```python
from build123d import *

# Parameters (mm, degrees)
F0_R     = 1.778
F1_DEPTH = 3.5
F2_DEPTH = 4


with BuildPart() as f1:
    # F0 (on Top) → F1 (new body)
    with BuildSketch(Plane.XY):
        with BuildLine():
            ThreePointArc((0, 5), (1.464466, 1.464466), (5, 0))
            Line((5, 0), (75, 0))
            Line((75, 0), (145, 0))
            ThreePointArc((145, 0), (148.535534, 1.464466), (150, 5))
            Line((150, 5), (150, 10))
            Line((150, 10), (150, 22.333333))
            Line((150, 22.333333), (150, 32.333333))
            Line((150, 32.333333), (150, 44.666667))
            Line((150, 44.666667), (150, 44.792384))
            Line((150, 44.792384), (150, 54.666667))
            Line((150, 54.666667), (150, 67))
            Line((150, 67), (150, 72))
            ThreePointArc((150, 72), (148.535534, 75.535534), (145, 77))
            Line((145, 77), (75, 77))
            Line((75, 77), (5, 77))
            ThreePointArc((5, 77), (1.464466, 75.535534), (0, 72))
            Line((0, 72), (0, 67))
            Line((0, 67), (0, 54.666667))
            Line((0, 54.666667), (0, 44.792384))
            Line((0, 44.792384), (0, 44.666667))
            Line((0, 44.666667), (0, 32.333333))
            Line((0, 32.333333), (0, 22.333333))
            Line((0, 22.333333), (0, 10))
            Line((0, 10), (0, 5))
        make_face()
        with Locations((7.5, 5)):
            Circle(F0_R, mode=Mode.SUBTRACT)
        with Locations((62, 5)):
            Circle(F0_R, mode=Mode.SUBTRACT)
        with BuildLine():
            Line((60.399714, 10), (18.611655, 10))
            ThreePointArc((18.611655, 10), (15.076121, 11.464466), (13.611655, 15))
            Line((13.611655, 15), (13.611655, 17.333333))
            ThreePointArc((13.611655, 17.333333), (15.076121, 20.868867), (18.611655, 22.333333))
            Line((18.611655, 22.333333), (60.399714, 22.333333))
            ThreePointArc((60.399714, 22.333333), (63.935248, 20.868867), (65.399714, 17.333333))
            Line((65.399714, 17.333333), (65.399714, 15))
            ThreePointArc((65.399714, 15), (63.935248, 11.464466), (60.399714, 10))
        make_face(mode=Mode.SUBTRACT)
        with Locations((7.5, 27.333333)):
            Circle(F0_R, mode=Mode.SUBTRACT)
        with Locations((62, 27.333333)):
            Circle(F0_R, mode=Mode.SUBTRACT)
        with Locations((88, 5)):
            Circle(F0_R, mode=Mode.SUBTRACT)
        with BuildLine():
            ThreePointArc((131.388345, 22.333333), (134.923879, 20.868867), (136.388345, 17.333333))
            Line((136.388345, 17.333333), (136.388345, 15))
            ThreePointArc((136.388345, 15), (134.923879, 11.464466), (131.388345, 10))
            Line((131.388345, 10), (89.600286, 10))
            ThreePointArc((89.600286, 10), (86.064752, 11.464466), (84.600286, 15))
            Line((84.600286, 15), (84.600286, 17.333333))
            ThreePointArc((84.600286, 17.333333), (86.064752, 20.868867), (89.600286, 22.333333))
            Line((89.600286, 22.333333), (131.388345, 22.333333))
        make_face(mode=Mode.SUBTRACT)
        with Locations((142.5, 5)):
            Circle(F0_R, mode=Mode.SUBTRACT)
        with Locations((88, 27.333333)):
            Circle(F0_R, mode=Mode.SUBTRACT)
        with Locations((142.5, 27.333333)):
            Circle(F0_R, mode=Mode.SUBTRACT)
        with Locations((7.5, 49.666667)):
            Circle(F0_R, mode=Mode.SUBTRACT)
        with BuildLine():
            Line((60.399714, 32.333333), (18.611655, 32.333333))
            ThreePointArc((18.611655, 32.333333), (15.076121, 33.797799), (13.611655, 37.333333))
            Line((13.611655, 37.333333), (13.611655, 39.792384))
            ThreePointArc((13.611655, 39.792384), (15.076121, 43.327917), (18.611655, 44.792384))
            Line((18.611655, 44.792384), (60.399714, 44.792384))
            ThreePointArc((60.399714, 44.792384), (63.935248, 43.327917), (65.399714, 39.792384))
            Line((65.399714, 39.792384), (65.399714, 37.333333))
            ThreePointArc((65.399714, 37.333333), (63.935248, 33.797799), (60.399714, 32.333333))
        make_face(mode=Mode.SUBTRACT)
        with Locations((62, 49.666667)):
            Circle(F0_R, mode=Mode.SUBTRACT)
        with Locations((7.5, 72)):
            Circle(F0_R, mode=Mode.SUBTRACT)
        with BuildLine():
            Line((60.399714, 54.666667), (18.611655, 54.666667))
            ThreePointArc((18.611655, 54.666667), (15.076121, 56.131133), (13.611655, 59.666667))
            Line((13.611655, 59.666667), (13.611655, 62))
            ThreePointArc((13.611655, 62), (15.076121, 65.535534), (18.611655, 67))
            Line((18.611655, 67), (60.399714, 67))
            ThreePointArc((60.399714, 67), (63.935248, 65.535534), (65.399714, 62))
            Line((65.399714, 62), (65.399714, 59.666667))
            ThreePointArc((65.399714, 59.666667), (63.935248, 56.131133), (60.399714, 54.666667))
        make_face(mode=Mode.SUBTRACT)
        with Locations((62, 72)):
            Circle(F0_R, mode=Mode.SUBTRACT)
        with BuildLine():
            Line((89.600286, 44.792384), (131.388345, 44.792384))
            ThreePointArc((131.388345, 44.792384), (134.923879, 43.327917), (136.388345, 39.792384))
            Line((136.388345, 39.792384), (136.388345, 37.333333))
            ThreePointArc((136.388345, 37.333333), (134.923879, 33.797799), (131.388345, 32.333333))
            Line((131.388345, 32.333333), (89.600286, 32.333333))
            ThreePointArc((89.600286, 32.333333), (86.064752, 33.797799), (84.600286, 37.333333))
            Line((84.600286, 37.333333), (84.600286, 39.792384))
            ThreePointArc((84.600286, 39.792384), (86.064752, 43.327917), (89.600286, 44.792384))
        make_face(mode=Mode.SUBTRACT)
        with Locations((88, 49.666667)):
            Circle(F0_R, mode=Mode.SUBTRACT)
        with Locations((142.5, 49.666667)):
            Circle(F0_R, mode=Mode.SUBTRACT)
        with BuildLine():
            ThreePointArc((131.388345, 67), (134.923879, 65.535534), (136.388345, 62))
            Line((136.388345, 62), (136.388345, 59.666667))
            ThreePointArc((136.388345, 59.666667), (134.923879, 56.131133), (131.388345, 54.666667))
            Line((131.388345, 54.666667), (89.600286, 54.666667))
            ThreePointArc((89.600286, 54.666667), (86.064752, 56.131133), (84.600286, 59.666667))
            Line((84.600286, 59.666667), (84.600286, 62))
            ThreePointArc((84.600286, 62), (86.064752, 65.535534), (89.600286, 67))
            Line((89.600286, 67), (131.388345, 67))
        make_face(mode=Mode.SUBTRACT)
        with Locations((88, 72)):
            Circle(F0_R, mode=Mode.SUBTRACT)
        with Locations((142.5, 72)):
            Circle(F0_R, mode=Mode.SUBTRACT)
    extrude(amount=F1_DEPTH)

    # F0 (on Top) → F2 (join)
    with BuildSketch(Plane.XY):
        with BuildLine():
            ThreePointArc((0, 5), (1.464466, 1.464466), (5, 0))
            Line((5, 0), (75, 0))
            Line((75, 0), (145, 0))
            ThreePointArc((145, 0), (148.535534, 1.464466), (150, 5))
            Line((150, 5), (150, 10))
            Line((150, 10), (150, 22.333333))
            Line((150, 22.333333), (150, 32.333333))
            Line((150, 32.333333), (150, 44.666667))
            Line((150, 44.666667), (150, 44.792384))
            Line((150, 44.792384), (150, 54.666667))
            Line((150, 54.666667), (150, 67))
            Line((150, 67), (150, 72))
            ThreePointArc((150, 72), (148.535534, 75.535534), (145, 77))
            Line((145, 77), (75, 77))
            Line((75, 77), (5, 77))
            ThreePointArc((5, 77), (1.464466, 75.535534), (0, 72))
            Line((0, 72), (0, 67))
            Line((0, 67), (0, 54.666667))
            Line((0, 54.666667), (0, 44.792384))
            Line((0, 44.792384), (0, 44.666667))
            Line((0, 44.666667), (0, 32.333333))
            Line((0, 32.333333), (0, 22.333333))
            Line((0, 22.333333), (0, 10))
            Line((0, 10), (0, 5))
        make_face()
        with Locations((7.5, 5)):
            Circle(F0_R, mode=Mode.SUBTRACT)
        with Locations((62, 5)):
            Circle(F0_R, mode=Mode.SUBTRACT)
        with BuildLine():
            Line((60.399714, 10), (18.611655, 10))
            ThreePointArc((18.611655, 10), (15.076121, 11.464466), (13.611655, 15))
            Line((13.611655, 15), (13.611655, 17.333333))
            ThreePointArc((13.611655, 17.333333), (15.076121, 20.868867), (18.611655, 22.333333))
            Line((18.611655, 22.333333), (60.399714, 22.333333))
            ThreePointArc((60.399714, 22.333333), (63.935248, 20.868867), (65.399714, 17.333333))
            Line((65.399714, 17.333333), (65.399714, 15))
            ThreePointArc((65.399714, 15), (63.935248, 11.464466), (60.399714, 10))
        make_face(mode=Mode.SUBTRACT)
        with Locations((7.5, 27.333333)):
            Circle(F0_R, mode=Mode.SUBTRACT)
        with Locations((62, 27.333333)):
            Circle(F0_R, mode=Mode.SUBTRACT)
        with Locations((88, 5)):
            Circle(F0_R, mode=Mode.SUBTRACT)
        with BuildLine():
            ThreePointArc((131.388345, 22.333333), (134.923879, 20.868867), (136.388345, 17.333333))
            Line((136.388345, 17.333333), (136.388345, 15))
            ThreePointArc((136.388345, 15), (134.923879, 11.464466), (131.388345, 10))
            Line((131.388345, 10), (89.600286, 10))
            ThreePointArc((89.600286, 10), (86.064752, 11.464466), (84.600286, 15))
            Line((84.600286, 15), (84.600286, 17.333333))
            ThreePointArc((84.600286, 17.333333), (86.064752, 20.868867), (89.600286, 22.333333))
            Line((89.600286, 22.333333), (131.388345, 22.333333))
        make_face(mode=Mode.SUBTRACT)
        with Locations((142.5, 5)):
            Circle(F0_R, mode=Mode.SUBTRACT)
        with Locations((88, 27.333333)):
            Circle(F0_R, mode=Mode.SUBTRACT)
        with Locations((142.5, 27.333333)):
            Circle(F0_R, mode=Mode.SUBTRACT)
        with Locations((7.5, 49.666667)):
            Circle(F0_R, mode=Mode.SUBTRACT)
        with BuildLine():
            Line((60.399714, 32.333333), (18.611655, 32.333333))
            ThreePointArc((18.611655, 32.333333), (15.076121, 33.797799), (13.611655, 37.333333))
            Line((13.611655, 37.333333), (13.611655, 39.792384))
            ThreePointArc((13.611655, 39.792384), (15.076121, 43.327917), (18.611655, 44.792384))
            Line((18.611655, 44.792384), (60.399714, 44.792384))
            ThreePointArc((60.399714, 44.792384), (63.935248, 43.327917), (65.399714, 39.792384))
            Line((65.399714, 39.792384), (65.399714, 37.333333))
            ThreePointArc((65.399714, 37.333333), (63.935248, 33.797799), (60.399714, 32.333333))
        make_face(mode=Mode.SUBTRACT)
        with Locations((62, 49.666667)):
            Circle(F0_R, mode=Mode.SUBTRACT)
        with Locations((7.5, 72)):
            Circle(F0_R, mode=Mode.SUBTRACT)
        with BuildLine():
            Line((60.399714, 54.666667), (18.611655, 54.666667))
            ThreePointArc((18.611655, 54.666667), (15.076121, 56.131133), (13.611655, 59.666667))
            Line((13.611655, 59.666667), (13.611655, 62))
            ThreePointArc((13.611655, 62), (15.076121, 65.535534), (18.611655, 67))
            Line((18.611655, 67), (60.399714, 67))
            ThreePointArc((60.399714, 67), (63.935248, 65.535534), (65.399714, 62))
            Line((65.399714, 62), (65.399714, 59.666667))
            ThreePointArc((65.399714, 59.666667), (63.935248, 56.131133), (60.399714, 54.666667))
        make_face(mode=Mode.SUBTRACT)
        with Locations((62, 72)):
            Circle(F0_R, mode=Mode.SUBTRACT)
        with BuildLine():
            Line((89.600286, 44.792384), (131.388345, 44.792384))
            ThreePointArc((131.388345, 44.792384), (134.923879, 43.327917), (136.388345, 39.792384))
            Line((136.388345, 39.792384), (136.388345, 37.333333))
            ThreePointArc((136.388345, 37.333333), (134.923879, 33.797799), (131.388345, 32.333333))
            Line((131.388345, 32.333333), (89.600286, 32.333333))
            ThreePointArc((89.600286, 32.333333), (86.064752, 33.797799), (84.600286, 37.333333))
            Line((84.600286, 37.333333), (84.600286, 39.792384))
            ThreePointArc((84.600286, 39.792384), (86.064752, 43.327917), (89.600286, 44.792384))
        make_face(mode=Mode.SUBTRACT)
        with Locations((88, 49.666667)):
            Circle(F0_R, mode=Mode.SUBTRACT)
        with Locations((142.5, 49.666667)):
            Circle(F0_R, mode=Mode.SUBTRACT)
        with BuildLine():
            ThreePointArc((131.388345, 67), (134.923879, 65.535534), (136.388345, 62))
            Line((136.388345, 62), (136.388345, 59.666667))
            ThreePointArc((136.388345, 59.666667), (134.923879, 56.131133), (131.388345, 54.666667))
            Line((131.388345, 54.666667), (89.600286, 54.666667))
            ThreePointArc((89.600286, 54.666667), (86.064752, 56.131133), (84.600286, 59.666667))
            Line((84.600286, 59.666667), (84.600286, 62))
            ThreePointArc((84.600286, 62), (86.064752, 65.535534), (89.600286, 67))
            Line((89.600286, 67), (131.388345, 67))
        make_face(mode=Mode.SUBTRACT)
        with Locations((88, 72)):
            Circle(F0_R, mode=Mode.SUBTRACT)
        with Locations((142.5, 72)):
            Circle(F0_R, mode=Mode.SUBTRACT)
    extrude(amount=F2_DEPTH)


solid = f1.part
```
The listing builds one solid part. Answer for the finished solid, in the listing's coordinates (mm). A direction names the side the tool comes from. Round coordinates to 2 decimals unless told otherwise and drop trailing zeros. Loops run counter-clockwise (first coordinate to the right, second up) from the corner with the lowest first, then second, coordinate; pieces in that order, holes last.
Q1. Section A-A, the plane x = 24 is taken. Determine the outline of the cut face in (y, z), then the cut area to 3 significant figures.
Q2. Which of the six approach directions +Z, -Z, +X, -X, +Y, -Y give full straight-line access (tool end or side, diameter ignored) to faces 1 (the face through (74, 0, 2)), 2 (the face through (86.026, 20.83, 1.972))?
Q3. Section B-B, the plane x = 142.5 is taken. Determine the outline of the cut face in (y, z).
Q4. Given pin 1 Ø5.5 at (x, y) = (88, 5) entering from +Z, flat-ended and moving along its own axis, determine where the tip first touches the part or whether it passes through.
Q5. Find the intervals of material crossed by line 1 (Y direction, x = 26, z = 2.6); line 2 (X direction, y = 72, z = 0.9); line 3 (X direction, y = 15, z = 2.35), in increasing order.
Q6. Section C-C, the plane y = 20.5 is taken. Determine the outline of the cut face in (x, z).
Q7. Section D-D, the plane x = 62 is taken. Count the separate pieces of the cut face and the enclosed holes in it, then the cut area to 3 significant figures.
Q8. For a pull along X with two mould halves and no side action, classify faces 3 (the face through (150, 38, 2)), 4 (the face through (15.04, 65.5, 1.97)), 5 (the face through (74, 39, 0)) as released by +X, released by -X, zero draft, split by the parting line, or undercut.
Completed:
1. outline: (0, 0) - (10, 0) - (10, 4) - (0, 4) - close; (22.33, 0) - (32.33, 0) - (32.33, 4) - (22.33, 4) - close; (44.79, 0) - (54.67, 0) - (54.67, 4) - (44.79, 4) - close; (67, 0) - (77, 0) - (77, 4) - (67, 4) - close
1. area: 159 mm2
2. face 1: +Z, -Z, +X, -X, -Y
2. face 2: +Z, -Z
3. outline: (0, 0) - (3.22, 0) - (3.22, 4) - (0, 4) - close; (6.78, 0) - (25.56, 0) - (25.56, 4) - (6.78, 4) - close; (29.11, 0) - (47.89, 0) - (47.89, 4) - (29.11, 4) - close; (51.44, 0) - (70.22, 0) - (70.22, 4) - (51.44, 4) - close; (73.78, 0) - (77, 0) - (77, 4) - (73.78, 4) - close
4. pin 1: stops at z = 4
5. line 1: y = 0 to 10, 22.33 to 32.33, 44.79 to 54.67, 67 to 77
5. line 2: x = 0 to 5.72, 9.28 to 60.22, 63.78 to 86.22, 89.78 to 140.72, 144.28 to 150
5. line 3: x = 0 to 13.61, 65.4 to 84.6, 136.39 to 150
6. outline: (0, 0) - (14.74, 0) - (14.74, 4) - (0, 4) - close; (64.27, 0) - (85.73, 0) - (85.73, 4) - (64.27, 4) - close; (135.26, 0) - (150, 0) - (150, 4) - (135.26, 4) - close
7. separate pieces: 8
7. enclosed holes: 0
7. area: 109 mm2
8. face 3: released by +X
8. face 4: undercut
8. face 5: zero draft
